Autodesk Inventor part; units mm, degrees
ref_plane "YZ Plane" through (0, 0, 0) normal (1, 0, 0) x (0, 1, 0)
ref_plane "XZ Plane" through (0, 0, 0) normal (0, 1, 0) x (-1, 0, 0)
ref_plane "XY Plane" through (0, 0, 0) normal (0, 0, 1) x (1, 0, 0)
sketch "Sketch2" plane through (0, 0, 0) normal (0, 0, 1) x (1, 0, 0)
  line L0 (0, 0) -> (20, 0)
  line L1 (20, 0) -> (20, 32)
  line L2 (20, 32) -> (0, 32)
  line L3 (0, 32) -> (0, 0)
  dimension "d0" = 20
  dimension "d1" = 32
extrude "Plate1" add sketch "Sketch2" along normal blind 0.92
sketch "Sketch3" plane through (19.08, 32, 0) normal (1, 0, 0) x (0, 1, 0)
  line L0 (-32, 0) -> (0, 0)
  line L1 (0, 0) -> (0, 27.8)
  line L2 (0, 27.8) -> (-32, 27.8)
  line L3 (-32, 27.8) -> (-32, 0)
edge flange "Flange1" height 27.8 angle 90 thickness 0.92 bend radius 0.92 thickness toward (1, 0, 0) relief tear relief width 0.92 relief depth 0.46 edges at (20, 16, 0.92) wall of the first edge with corners at (19.08, 0, 0) (19.08, 32, 0) (19.08, 32, 27.8) (19.08, 0, 27.8)
bend "Bend1"
corner "Corner1"
sketch "Sketch4" plane through (20, 32, 26.88) normal (0, 0, 1) x (1, 0, 0)
  line L0 (0, -32) -> (0, 0)
  line L1 (0, 0) -> (-15, 0)
  line L2 (-15, 0) -> (-15, -32)
  line L3 (-15, -32) -> (0, -32)
edge flange "Flange2" height 15 angle 90 thickness 0.92 bend radius 0.92 thickness toward (0, 0, 1) relief tear relief width 0.92 relief depth 0.46 edges at (19.08, 16, 27.8) wall of the first edge with corners at (20, 0, 26.88) (20, 32, 26.88) (5, 32, 26.88) (5, 0, 26.88)
bend "Bend2"
corner "Corner2"
fillet "Fillet2" radius 2 4 edges at (0, 0, 0.46) (5, 32, 27.34) (5, 0, 27.34) (0, 32, 0.46)
sketch "Sketch5" plane through (0, 0, 0) normal (0, 0, -1) x (-1, 0, 0)
  line L0 (-20, 0) -> (-20, 32)
  line L1 (-18.16, 32) -> (-2, 32)
  line L2 (0, 30) -> (0, 2)
  line L3 (-2, 0) -> (-18.16, 0)
  point P0 (0, 0)
  point P1 (-15.15, 27.1)
  point P2 (-4.85, 4.9)
  dimension "d35" = 4.85
  dimension "d36" = 4.9
  dimension "d37" = 4.9
  dimension "d38" = 4.85
hole "Hole1" at (15.15, 27.1, 0) at (4.85, 4.9, 0) direction (0, 0, 1) diameter 2.459 depth 2 tip angle 137
sketch "Sketch6" plane through (18.16, 0, 27.8) normal (0, 0, 1) x (1, 0, 0)
  line L0 (-11.16, 32) -> (0, 32)
  line L1 (0, 0) -> (-11.16, 0)
  line L2 (-13.16, 2) -> (-13.16, 30)
  point P0 (-18.16, 0)
  point P1 (-5.66, 24)
  point P2 (-5.66, 8)
  dimension "d46" = 8
  dimension "d47" = 8
  dimension "d48" = 7.5
  dimension "d49" = 7.5
hole "Hole2" at (12.5, 24, 27.8) at (12.5, 8, 27.8) direction (0, 0, -1) diameter 4.134 depth 2 tip angle 137
equation "\"d2\" = Thickness"
equation "\"d3\" = BendReliefWidth"
equation "\"d4\" = BendReliefDepth"
equation "\"d5\" = MinimumRemnant"
equation "\"d6\" = TransitionRadius"
equation "\"d9\" = BendRadius"
equation "\"d10\" = CornerReliefSize"
equation "\"d11\" = GapSize"
equation "\"d12\" = JacobiRadiusSize"
equation "\"d13\" = BendReliefWidth"
equation "\"d14\" = BendReliefDepth"
equation "\"d15\" = MinimumRemnant"
equation "\"d16\" = TransitionRadius"
equation "\"d19\" = BendRadius"
equation "\"d20\" = CornerReliefSize"
equation "\"d21\" = GapSize"
equation "\"d22\" = JacobiRadiusSize"
equation "\"BendRadius\" = Thickness"
equation "\"BendReliefWidth\" = Thickness"
equation "\"BendReliefDepth\" = 0.5 * Thickness"
equation "\"CornerReliefSize\" = 4 * Thickness"
equation "\"MinimumRemnant\" = 2 * Thickness"
equation "\"TransitionRadius\" = BendRadius"
equation "\"JacobiRadiusSize\" = BendRadius"
equation "\"GapSize\" = Thickness"
properties part number "Soporte final de carrera" material "Steel AISI 1006 85 HR"
Source: CAD feature listing. Evaluate the final solid. Frame: model axes, mm. A direction names the side the tool comes from. Coordinates: 2 decimals unless noted, no trailing zeros. Order: outer loops, then holes, each group sorted by start corner. A loop starts at its lowest first (then second) coordinate and runs counter-clockwise, first axis right, second up. Notation, with made-up numbers: M 30.25,-6.75 L 49.25,-6.75 A22 cw 49.25,24.25 Z; hole C -5.5,70.25 d8. An arc over 180 degrees is marked long. Write each question's results on one line, items separated by ' | '. Start each with the question number.
1) Section query A-A (x = 12.5). Return the cut outline in (y, z), plus the area to 3 significant figures.
2) Contact query for flat-ended pins moving along their axis: pin 1 Ø0.5 at (y, z) = (17.5, 27) entering from -X; pin 2 Ø6 at (y, z) = (11.5, 7) entering from -X. Output: stop coordinate, or through.
3) Section query B-B (y = 4.9). Return the cut outline in (x, z), plus the area to 3 significant figures.
4) Section query D-D (y = 12). Return the cut outline in (x, z).
5) Draft query along Z for faces 5 (the face through (5.57, 0.6, 27.35)), 6 (the face through (19.08, 16, 14)), 7 (the face through (9, 16, 0)), 8 (the face through (18.8, 16.22, 26.62)). Return one class per face: released by +Z, released by -Z, zero draft, split by the parting line, or undercut.
6) Section query C-C (x = 7.5). Return the cut outline in (y, z).
7) Access query for faces 1 (the face through (18.82, 16.22, 1.2)), 2 (the face through (14.518, 8.448, 27.334)), 3 (the face through (5.94, 5.47, 0.47)), 4 (the face through (5, 16.2, 27.3)). Directions: +Z, -Z, +X, -X, +Y, -Y. A direction counts if a zero-diameter tool reaches every point of the face in a straight line with its end or side. Return the directions, or none.
8) Line query: line 1 (Y direction, x = 12.5, z = 27.6); line 2 (Z direction, x = 17.5, y = 5.5); line 3 (X direction, y = 29, z = 17.75). Output: solid intervals per line, ascending. Write a range as from..to.
Answers:
1) outline: M 0,0 L 32,0 L 32,0.92 L 0,0.92 Z; M 0,26.88 L 5.93,26.88 L 5.93,27.8 L 0,27.8 Z; M 10.07,26.88 L 21.93,26.88 L 21.93,27.8 L 10.07,27.8 Z; M 26.07,26.88 L 32,26.88 L 32,27.8 L 26.07,27.8 Z | area: 51.3 mm^2
2) pin 1: stops at x = 5 | pin 2: stops at x = 19.08
3) outline: M 0,0 L 3.62,0 L 3.62,0.92 L 0,0.92 Z; M 5,26.88 L 18.16,26.88 A0.92 cw 19.08,25.96 L 19.08,1.84 A0.92 cw 18.16,0.92 L 6.08,0.92 L 6.08,0 L 18.16,0 A1.84 ccw 20,1.84 L 20,25.96 A1.84 ccw 18.16,27.8 L 5,27.8 Z | area: 52.7 mm^2
4) outline: M 0,0 L 18.16,0 A1.84 ccw 20,1.84 L 20,25.96 A1.84 ccw 18.16,27.8 L 5,27.8 L 5,26.88 L 18.16,26.88 A0.92 cw 19.08,25.96 L 19.08,1.84 A0.92 cw 18.16,0.92 L 0,0.92 Z
5) face 5: zero draft | face 6: undercut | face 7: released by -Z | face 8: undercut
6) outline: M 0,0 L 32,0 L 32,0.92 L 0,0.92 Z; M 0,26.88 L 32,26.88 L 32,27.8 L 0,27.8 Z
7) face 1: -X, +Y, -Y | face 2: +Z | face 3: -Z | face 4: +Z, -X, +Y, -Y
8) line 1: y = 0..5.93, 10.07..21.93, 26.07..32 | line 2: z = 0..0.92, 26.88..27.8 | line 3: x = 19.08..20
